Autodesk Inventor part; units mm, degrees
ref_plane "YZ Plane" through (0, 0, 0) normal (1, 0, 0) x (0, 1, 0)
ref_plane "XZ Plane" through (0, 0, 0) normal (0, 1, 0) x (-1, 0, 0)
ref_plane "XY Plane" through (0, 0, 0) normal (0, 0, 1) x (1, 0, 0)
sketch "Boceto1" plane through (0, 0, 0) normal (0, 0, 1) x (1, 0, 0)
  line L0 (-40, 40) -> (40, 40)
  line L1 (40, 40) -> (40, -40)
  line L2 (40, -40) -> (-40, -40)
  line L3 (-40, -40) -> (-40, 40)
  line L4 (-40, 40) -> (40, -40) construction
  line L5 (40, 40) -> (-40, -40) construction
  point P0 (0, 0)
  dimension "d0" = 80
  dimension "d1" = 80
extrude "Extrusión1" add sketch "Boceto1" along normal blind 50
sketch "Boceto2" plane through (0, 0, 50) normal (0, 0, 1) x (1, 0, 0)
  circle A0 centre (0, 0) radius 25
  circle A1 centre (0, 0) radius 20
  dimension "d4" = 50
  dimension "d5" = 5
extrude "Extrusión2" add sketch "Boceto2" along normal blind 50
sketch "Boceto3" plane through (0, 0, 0) normal (0, 0, -1) x (-1, 0, 0)
  line L0 (-40, 40) -> (40, 40)
  line L1 (40, 40) -> (40, -40)
  line L2 (-40, 40) -> (40, 40)
  line L3 (40, 40) -> (40, -40)
  line L4 (40, -40) -> (-40, -40)
  line L5 (-40, -40) -> (-40, 40)
  line L6 (-35, -36.4247) -> (35, 36.4247) construction
  line L7 (35, -36.4247) -> (-35, 36.4247) construction
  line L8 (-35, 36.4247) -> (-37.5, 36.4247)
  line L9 (-40, 36.4247) -> (-40, 40)
  line L10 (-40, 40) -> (-35, 40)
  line L11 (-35, 40) -> (-35, 38.9247)
  arc A0 (-35.0145, 36.4247) -> (-35.0108, 36.4359) centre (-35.2551, 36.5094) ccw
  circle A1 centre (-35, 36.4247) radius 2.5
  circle A2 centre (35, 36.4247) radius 2.5
  circle A3 centre (-35, -36.4247) radius 2.5
  circle A4 centre (35, -36.4247) radius 2.5
  line L12 (35, 36.4247) -> (32.5, 36.4247)
  line L13 (-32.5, 36.4247) -> (-35, 36.4247)
  line L14 (35, -36.4247) -> (35, -33.9247)
  line L15 (35, 33.9247) -> (35, 36.4247)
  line L16 (-35, 36.4247) -> (-35, 33.9247)
  line L17 (-35, -33.9247) -> (-35, -36.4247)
  line L18 (-35, -36.4247) -> (-32.5, -36.4247)
  line L19 (32.5, -36.4247) -> (35, -36.4247)
  point P0 (0, 0)
  point P1 (-38.2122, 38.2122)
  dimension "d9" = 70
sketch "Boceto4" plane through (0, 0, 0) normal (0, 0, -1) x (-1, 0, 0)
  point P0 (0, 0)
extrude "Extrusión3" cut sketch "Boceto3" against normal blind 50 contours A1 L13 L8 | A1 L16 L13 | L8 L16 A1 | A2 L15 L12 | L12 L15 A2 | L18 L17 A3 | A3 L17 L18 | A4 L19 L14 | L14 L19 A4
thread "Rosca1"
thread "Rosca2"
thread "Rosca3"
thread "Rosca4"
fillet "Empalme1" radius 2 4 edges at (0, -40, 50) (40, 0, 50) (0, 40, 50) (-40, 0, 50)
thread "Rosca5"
sketch "Boceto5" plane through (0, 0, 50) normal (0, 0, 1) x (1, 0, 0)
  circle A0 centre (0, 0) radius 20
extrude "Extrusión4" add sketch "Boceto5" along normal blind 20
properties part number "Lab 1"
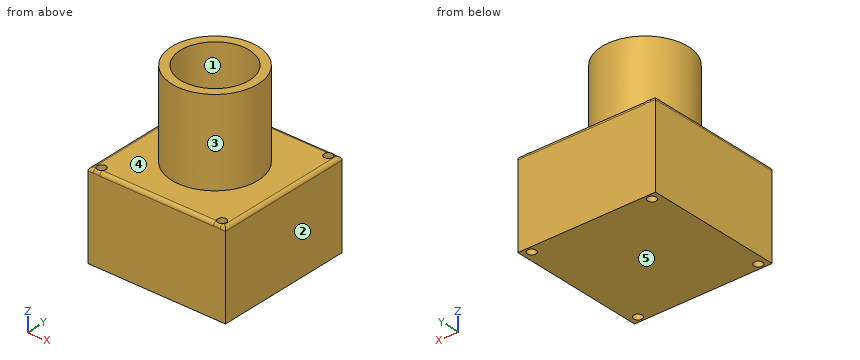
Geometry: final body of the model. Coordinates: model frame, mm. Face numbers are marked on the shaded views. A direction names the side the tool comes from. Give positions to 0.01 mm unless a question says otherwise; leave off trailing zeros. Write each loop counter-clockwise with the first axis right and the second up, starting at its lowest first coordinate (ties: lowest second). Pieces come first, ordered by that corner, then holes. Notation, with made-up numbers: (48, 74.5) -> (57, 74.5) arc R18 cw to (57, 109.5) -> close; hole circle Ø9 at (-9.5, 43.5). An arc over 180 degrees is marked (long way). Answer in a Markdown table with one row per item.
(1) Section query C-C on x = 35. State how many separate pieces and enclosed holes the cut face has, then the cut area to 3 significant figures.
Answers below:
| item | result |
|---|---|
| separate pieces | 3 |
| enclosed holes | 0 |
| area | 3,500 mm^2 |
(2) Section query D-D on y = 31. Return loops of the section in (x, z), then the cut area to 3 significant figures.
Answers below:
| item | result |
|---|---|
| outline | (-40, 0) -> (40, 0) -> (40, 48) arc R2 ccw to (38, 50) -> (-38, 50) arc R2 ccw to (-40, 48) -> close |
| area | 4,000 mm^2 |
(3) Pin query (flat end, axial travel): pin 1 (12 mm diameter, centred on x = 9, y = -0.5, fed in from +Z); pin 2 (12 mm diameter, centred on x = 24.5, y = -28, fed in from +Z); pin 3 (12 mm diameter, centred on x = -17, y = -24, fed in from -Z); pin 4 (4 mm diameter, centred on x = 21.5, z = 61.5, fed in from -Y). Return the tip coordinate at first contact, or that it passes through.
Answers below:
| item | result |
|---|---|
| pin 1 | z = 70 |
| pin 2 | z = 50 |
| pin 3 | z = 0 |
| pin 4 | y = -15.64 |
(4) Draft query along X for the marked faces 1, 2 and 3. Return one class per face: +X half, -X half, draft (parallel to the pull), parting line (faces both ways), or undercut.
Answers below:
| item | result |
|---|---|
| face 1 | undercut |
| face 2 | +X half |
| face 3 | parting line |
(5) Section query A-A on y = 0. Return loops of the section in (x, z).
Answers below:
| item | result |
|---|---|
| outline | (-40, 0) -> (40, 0) -> (40, 48) arc R2 ccw to (38, 50) -> (25, 50) -> (25, 100) -> (20, 100) -> (20, 70) -> (-20, 70) -> (-20, 100) -> (-25, 100) -> (-25, 50) -> (-38, 50) arc R2 ccw to (-40, 48) -> close |
(6) Ray query, line 1 along Y through (x, z) = (35, 20); line 2 along Y through (x, z) = (-34.5, 16); line 3 along X through (y, z) = (-0.5, 85) (3 decimals). Return the intervals inside material, ascending. Write a range as [from, to].
Answers below:
| item | result |
|---|---|
| line 1 | [-40, -38.92], [-33.92, 33.92], [38.92, 40] |
| line 2 | [-40, -38.87], [-33.98, 33.98], [38.87, 40] |
| line 3 | [-24.995, -19.994], [19.994, 24.995] |
(7) Set-up query: the marked faces 4 and 5. Return all of +Z, -Z, +X, -X, +Y, -Y with unobstructed straight access to the full face (end or side cutting, diameter ignored); none if empty.
Answers below:
| item | result |
|---|---|
| face 4 | +Z |
| face 5 | -Z, +X, -X, +Y, -Y |
